Work out the finished part from the listing and answer in its coordinate system (mm). Face numbers are marked on the shaded views. A direction names the side the tool comes from. Give positions to 0.01 mm unless a question says otherwise; leave off trailing zeros. Order: outer loops, then holes, each group sorted by start corner. A loop starts at its lowest first (then second) coordinate and runs counter-clockwise, first axis right, second up. Notation, with made-up numbers: (74, -38) -> (114, -38) arc R13 ccw to (114, -17) -> close; hole circle Ø10 at (70, 26.5). An arc over 180 degrees is marked (long way). Use a Markdown table: item, result. Add a question column.
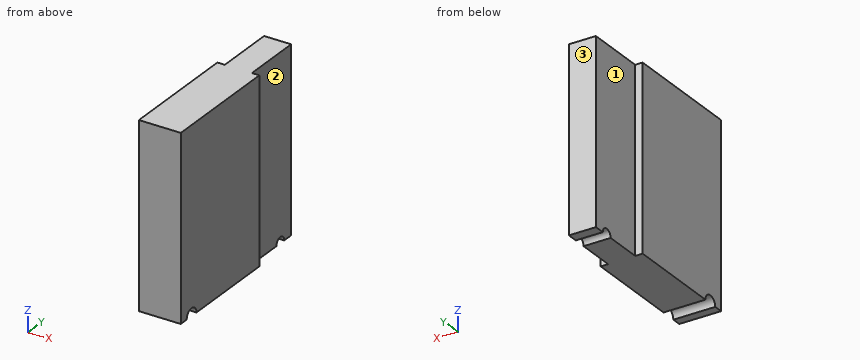
```python
from build123d import *

# Parameters (mm, degrees)
SKETCH_W      = 6.9
SKETCH_H      = 20
PAD_DEPTH     = 30
SKETCH001_W   = 4.45
SKETCH001_H   = 10
PAD001_DEPTH  = 30
SKETCH002_R   = 1
SKETCH002_R_2 = 1.25
POCKET_DEPTH  = 20


with BuildPart() as part:
    # Sketch → Pad (new body)
    with BuildSketch(Plane.XY):
        Rectangle(SKETCH_W, SKETCH_H)
    extrude(amount=PAD_DEPTH)

    # Sketch001 → Pad001 (join)
    with BuildSketch(Plane.XY):
        with Locations((0, 15)):
            Rectangle(SKETCH001_W, SKETCH001_H)
    extrude(amount=PAD001_DEPTH)

    # Sketch002 (on Face4 of Pad001) → Pocket (cut, symmetric)
    with BuildSketch(Plane.YZ.offset(2.225)):
        with Locations((17.25, 0)):
            Circle(SKETCH002_R)
        with Locations((-7.25, 0)):
            Circle(SKETCH002_R_2)
    extrude(amount=POCKET_DEPTH, both=True, mode=Mode.SUBTRACT)


solid = part.part
```
1) Flat-ended cylindrical pins translate along their axes: pin 1 (0.6 mm diameter, centred on x = 3, z = 11.5, fed in from +Y); pin 2 (2 mm diameter, centred on x = 2.5, y = 16, fed in from -Z). Find the tip coordinate at first contact, or state that the pin passes through.
2) The part is cut by section A-A, the plane z = 28.25. Determine the outline of the cut face in (x, y) (3 decimals), then the cut area to 4 significant figures.
3) Straight lines are drawn through the part: line 1 (Y direction, x = 2.5, z = 3.5); line 2 (X direction, y = 16.5, z = 28.5) (3 decimals); line 3 (Z direction, x = 0.5, y = -8). For each, find the intervals that lie inside material, in ascending order.
4) The part is cut by section C-C, the plane y = 13.25. Determine the outline of the cut face in (x, z) (3 decimals), then the cut area to 4 significant figures.
5) Which of the six approach directions +Z, -Z, +X, -X, +Y, -Y give full straight-line access (tool end or side, diameter ignored) to the marked faces 1, 2 and 3?
6) The part is cut by section B-B, the plane y = -7.25. Determine the outline of the cut face in (x, z), then the cut area to 3 significant figures.
A:
| question | item | result |
|---|---|---|
| 1 | pin 1 | y = 10 |
| 1 | pin 2 | z = 0 |
| 2 | outline | (-3.45, -10) -> (3.45, -10) -> (3.45, 10) -> (2.225, 10) -> (2.225, 20) -> (-2.225, 20) -> (-2.225, 10) -> (-3.45, 10) -> close |
| 2 | area | 182.5 mm^2 |
| 3 | line 1 | -10 to 10 |
| 3 | line 2 | -2.225 to 2.225 |
| 3 | line 3 | 1 to 30 |
| 4 | outline | (-2.225, 0) -> (2.225, 0) -> (2.225, 30) -> (-2.225, 30) -> close |
| 4 | area | 133.5 mm^2 |
| 5 | face 1 | +Z, -Z, -X, +Y |
| 5 | face 2 | +Z, -Z, +X, +Y |
| 5 | face 3 | +Z, -Z, +X, -X, +Y |
| 6 | outline | (-3.45, 1.25) -> (3.45, 1.25) -> (3.45, 30) -> (-3.45, 30) -> close |
| 6 | area | 198 mm^2 |
